Geometry check sheet. Reference: the model listing, model coordinates, mm. Face numbers are marked on the shaded views. A direction names the side the tool comes from. Give positions to 0.01 mm unless a question says otherwise; leave off trailing zeros. Write each loop counter-clockwise with the first axis right and the second up, starting at its lowest first coordinate (ties: lowest second). Pieces come first, ordered by that corner, then holes. Notation, with made-up numbers: (17.25, 50.25) - (63.25, 50.25) arc R26 ccw to (63.25, 88.25) - close; hole circle Ø8 at (21.5, 56). An arc over 180 degrees is marked (long way). Write item = value, one per line. Start each with the question number.
(1) Section check D-D, the plane x = -5.25. Enter the section's corners in (y, z).
(2) Draft check along Y on the marked faces 3, 4 and 5. Enter one of: pulls with the +Y half, pulls with the -Y half, needs draft (parallel to the pull), parting line crosses it, or undercut.
(3) Thickness scan on L1, parallel to Y at x = 0, z = 5.25; L2, parallel to Z at x = 4.75, y = -0.25; L3, parallel to Y at x = 2, z = 3. Record the ranges inside material, lowest first.
(4) Section check B-B, the plane z = 2.5. Enter the section's corners in (x, y), plus the area to 3 significant figures.
(5) Section check C-C, the plane z = -16.5. Enter the section's corners in (x, y).
(6) Depth check by flat-ended pin: pin 1 Ø8 at (y, z) = (-2.5, 0.5) entering from +X; pin 2 Ø5 at (x, z) = (-3, 1.5) entering from +Y; pin 3 Ø8 at (x, z) = (1, -14.5) entering from -Y; pin 4 Ø3 at (y, z) = (2, 0.5) entering from -X. Enter the tip coordinate at first touch or a pass-through.
(7) Access from +Z, -Z, +X, -X, +Y, -Y to the whole of each face (thin tool, end or side, straight path). Record for the marked faces 1 and 2.
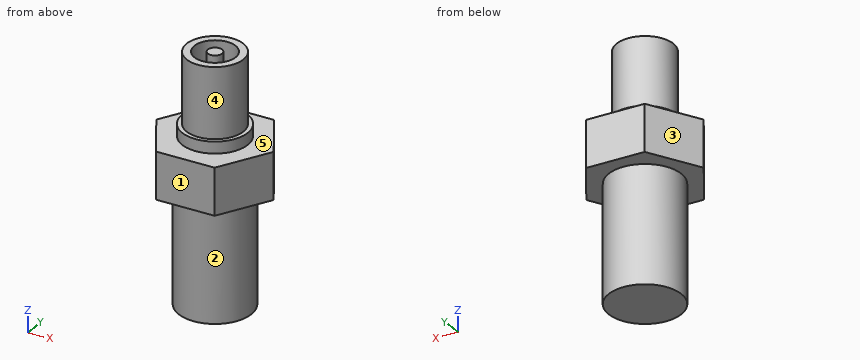
```python
from build123d import *

# Parameters (mm, degrees)
SKETCH1_R          = 3.85
EXTRUDE1_DEPTH     = 9.525
SKETCH2_R          = 4.445
EXTRUDE2_DEPTH     = 1.5875
EXTRUDE3_DEPTH     = 6.35
SKETCH4_R          = 4.9276
EXTRUDE4_DEPTH     = 15.875
SKETCH5_R          = 2.80042078
SKETCH5_R_2        = 0.97787642
CUT_EXTRUDE1_DEPTH = 9.525


with BuildPart() as part:
    # Sketch1 → Extrude1 (new body)
    with BuildSketch(Plane.XY):
        Circle(SKETCH1_R)
    extrude(amount=EXTRUDE1_DEPTH)

    # Sketch2 → Extrude2 (add)
    with BuildSketch(Plane(origin=(0, 0, 0), x_dir=(-1, 0, 0), z_dir=(0, 0, -1))):
        Circle(SKETCH2_R)
    extrude(amount=EXTRUDE2_DEPTH)

    # Sketch3 → Extrude3 (add)
    with BuildSketch(Plane(origin=(0, 0, -1.5875), x_dir=(-1, 0, 0), z_dir=(0, 0, -1))):
        Polygon((-3.959468146, 6.858), (3.959468146, 6.858), (7.918936292, 0), (3.959468146, -6.858), (-3.959468146, -6.858), (-7.918936292, 0), align=None)
    extrude(amount=EXTRUDE3_DEPTH)

    # Sketch4 → Extrude4 (add)
    with BuildSketch(Plane(origin=(0, 0, -7.9375), x_dir=(-1, 0, 0), z_dir=(0, 0, -1))):
        Circle(SKETCH4_R)
    extrude(amount=EXTRUDE4_DEPTH)

    # Sketch5 → Cut-Extrude1 (cut)
    with BuildSketch(Plane.XY.offset(9.525)):
        Circle(SKETCH5_R)
        Circle(SKETCH5_R_2, mode=Mode.SUBTRACT)
    extrude(amount=-CUT_EXTRUDE1_DEPTH, mode=Mode.SUBTRACT)


solid = part.part
```
Model answer:
q1.outline = (-4.62, -7.94) - (4.62, -7.94) - (4.62, -1.59) - (-4.62, -1.59) - close
q2.face_3 = pulls with the +Y half
q2.face_4 = parting line crosses it
q2.face_5 = needs draft
q3.L1 = -3.85 to -2.8, -0.98 to 0.98, 2.8 to 3.85
q3.L2 = -23.81 to -1.59
q3.L3 = -3.29 to -1.96, 1.96 to 3.29
q4.outline = circle Ø7.7 at (0, 0); circle Ø1.96 at (0, 0); hole circle Ø5.6 at (0, 0)
q4.area = 24.9 mm²
q5.outline = circle Ø9.86 at (0, 0)
q6.pin_1 = 7.92
q6.pin_2 = 4.33
q6.pin_3 = -4.93
q6.pin_4 = -4.41
q7.face_1 = +Z, -Z, +X, -X, -Y
q7.face_2 = -Z
